Build history of the part. All positions in model axes, mm. Face numbers are marked on the shaded views. A direction names the side the tool comes from. Give positions to 0.01 mm unless a question says otherwise; leave off trailing zeros. Write each loop counter-clockwise with the first axis right and the second up, starting at its lowest first coordinate (ties: lowest second). Pieces come first, ordered by that corner, then holes. Notation, with made-up numbers: (54.5, -18.5) -> (100.5, -18.5) arc R10 ccw to (100.5, -1.5) -> close; hole circle Ø7 at (-21, 83). An arc over 180 degrees is marked (long way). Put each result on its own line as item: value. Start each with the question number.
Item 1: Slice it at C-C, the plane x = 53. List the corners of the cut face in (y, z) (3 decimals), plus the area to 3 significant figures.
Item 2: Slice it at D-D, the plane y = -36. List the corners of the cut face in (x, z) (3 decimals).
Item 3: Flat gauge pins, fed straight in: pin 1 Ø12 at (x, z) = (9, 7) entering from -Y; pin 2 Ø2.5 at (y, z) = (-28, 3) entering from +X; pin 3 Ø5 at (y, z) = (-9, 19) entering from +X; pin 4 Ø5 at (x, y) = (22.5, -36) entering from +Z. Where does each tip first touch, or does it go through?
Item 4: Drill centre lines: line 1 along X through (y, z) = (-11, 12); line 2 along Z through (x, y) = (-19.5, -40) (3 decimals); line 3 along X through (y, z) = (-35, -15.5). Where is each one in solid material? Low to high.
Item 5: Two-plate mould, pull along Z, no slides. Class the marked faces 6, 7, 8 and 9: pulls with the +Z half, pulls with the -Z half, needs draft (parallel to the pull), parting line crosses it, or undercut.
Item 6: Slice it at B-B, the plane y = -11. List the corners of the cut face in (x, z) (1 decimal), plus the area to 3 significant figures.
Item 7: Slice it at A-A, the plane z = 12.7. List the corners of the cut face in (x, y) (1 decimal), plus the area to 3 significant figures.
Item 8: Tool access for the marked faces 1, 2, 3, 4 and 5: list every direction of +Z, -Z, +X, -X, +Y, -Y with a clear straight run to the whole face (end or side of a thin tool).
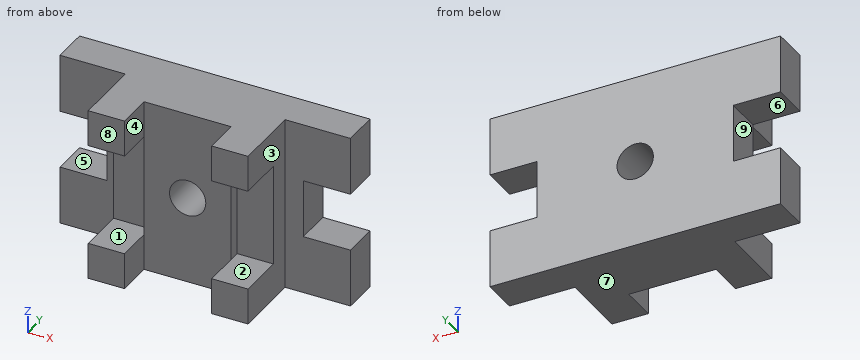
```python
from build123d import *

# Parameters (mm, degrees)
F1_DEPTH = 15.875
F2_DEPTH = 46.0375
F0_R     = 7.9375
F3_DEPTH = 30.1625
F4_DEPTH = 25.4


with BuildPart() as f1:
    # F0 (on Front) → F1 (new body)
    with BuildSketch(Plane.XZ):
        Polygon((-28.1177360594, 50.8), (-56.6927360594, 50.8), (-56.6927360594, 25.4), (-36.0552360594, 25.4), (-36.0552360594, 0), (-56.6927360594, 0), (-56.6927360594, -25.4), (-28.1177360594, -25.4), (-28.1177360594, -9.525), (-28.1177360594, 34.925), align=None)
    extrude(amount=F1_DEPTH)

    # F0 (on Front) → F2 (join)
    with BuildSketch(Plane.XZ):
        Polygon((-12.2427360594, 50.8), (-28.1177360594, 50.8), (-28.1177360594, 34.925), (-20.1802360594, 34.925), (-12.2427360594, 34.925), align=None)
        Polygon((-20.1802360594, -9.525), (-28.1177360594, -9.525), (-28.1177360594, -25.4), (-12.2427360594, -25.4), (-12.2427360594, -9.525), align=None)
    extrude(amount=F2_DEPTH)



with BuildPart() as f1b:
    # F0 (on Front) → F1, piece 2 (new body)
    with BuildSketch(Plane.XZ):
        Polygon((70.3072639406, 50.8), (41.7322639406, 50.8), (41.7322639406, 34.925), (41.7322639406, -9.525), (41.7322639406, -25.4), (70.3072639406, -25.4), (70.3072639406, 0), (49.6697639406, 0), (49.6697639406, 25.4), (70.3072639406, 25.4), align=None)
    extrude(amount=F1_DEPTH)

    # F0 (on Front) → F2, piece 2 (join)
    with BuildSketch(Plane.XZ):
        Polygon((41.7322639406, 50.8), (25.8572639406, 50.8), (25.8572639406, 34.925), (33.7947639406, 34.925), (41.7322639406, 34.925), align=None)
        Polygon((33.7947639406, -9.525), (25.8572639406, -9.525), (25.8572639406, -25.4), (41.7322639406, -25.4), (41.7322639406, -9.525), align=None)
    extrude(amount=F2_DEPTH)


with BuildPart() as f1_1:
    add(f1.part)

    add(f1b.part)  # F3 merges F1b
    # F0 (on Front) → F3 (join)
    with BuildSketch(Plane.XZ):
        Polygon((25.8572639406, 50.8), (-12.2427360594, 50.8), (-12.2427360594, 34.925), (-12.2427360594, -9.525), (-12.2427360594, -25.4), (25.8572639406, -25.4), (25.8572639406, -9.525), (25.8572639406, 34.925), align=None)
        with Locations((6.8072639406, 12.7)):
            Circle(F0_R, mode=Mode.SUBTRACT)
    extrude(amount=F3_DEPTH)

    # F0 (on Front) → F4 (join)
    with BuildSketch(Plane.XZ):
        Polygon((-20.1802360594, 34.925), (-28.1177360594, 34.925), (-28.1177360594, -9.525), (-20.1802360594, -9.525), (-12.2427360594, -9.525), (-12.2427360594, 34.925), align=None)
        Polygon((33.7947639406, 34.925), (25.8572639406, 34.925), (25.8572639406, -9.525), (33.7947639406, -9.525), (41.7322639406, -9.525), (41.7322639406, 34.925), align=None)
    extrude(amount=F4_DEPTH)


solid = f1_1.part
```
Values follow:
1. outline: (-15.875, -25.4) -> (0, -25.4) -> (0, 0) -> (-15.875, 0) -> close; (-15.875, 25.4) -> (0, 25.4) -> (0, 50.8) -> (-15.875, 50.8) -> close
1. area: 806 mm2
2. outline: (-28.118, -25.4) -> (-12.243, -25.4) -> (-12.243, -9.525) -> (-28.118, -9.525) -> close; (-28.118, 34.925) -> (-12.243, 34.925) -> (-12.243, 50.8) -> (-28.118, 50.8) -> close; (25.857, -25.4) -> (41.732, -25.4) -> (41.732, -9.525) -> (25.857, -9.525) -> close; (25.857, 34.925) -> (41.732, 34.925) -> (41.732, 50.8) -> (25.857, 50.8) -> close
3. pin 1: y = -30.16
3. pin 2: x = 25.86
3. pin 3: x = 49.67
3. pin 4: through
4. line 1: -36.06 to -1.1, 14.71 to 49.67
4. line 2: -25.4 to -9.525, 34.925 to 50.8
4. line 3: -28.12 to -12.24, 25.86 to 41.73
5. face 6: undercut
5. face 7: pulls with the -Z half
5. face 8: needs draft
5. face 9: undercut
6. outline: (-56.7, -25.4) -> (70.3, -25.4) -> (70.3, 0) -> (49.7, 0) -> (49.7, 25.4) -> (70.3, 25.4) -> (70.3, 50.8) -> (-56.7, 50.8) -> (-56.7, 25.4) -> (-36.1, 25.4) -> (-36.1, 0) -> (-56.7, 0) -> close; hole circle Ø15.9 at (6.8, 12.7)
6. area: 8,430 mm2
7. outline: (-36.1, -15.9) -> (-28.1, -15.9) -> (-28.1, -25.4) -> (-12.2, -25.4) -> (-12.2, -30.2) -> (-1.1, -30.2) -> (-1.1, 0) -> (-36.1, 0) -> close; (14.7, -30.2) -> (25.9, -30.2) -> (25.9, -25.4) -> (41.7, -25.4) -> (41.7, -15.9) -> (49.7, -15.9) -> (49.7, 0) -> (14.7, 0) -> close
7. area: 1,730 mm2
8. face 1: -X, -Y
8. face 2: +X, -Y
8. face 3: +Z, -Z, +X, -Y
8. face 4: +Z, -Z, -Y
8. face 5: -X, +Y, -Y
